from build123d import *

# Parameters (mm, degrees)
SKETCH039_W       = 155
SKETCH039_H       = 187
SKETCH039_R       = 65
PAD004_DEPTH      = 2
PAD005_DEPTH      = 37
SKETCH041_R       = 66
SKETCH041_R_2     = 65
PAD006_DEPTH      = 33
PAD007_DEPTH      = 176
PAD012_DEPTH      = 73.5
PAD012_DEPTH_BACK = 73.5
SKETCH054_W       = 2
SKETCH054_H       = 130
POCKET013_DEPTH   = 2
SKETCH067_R       = 10
POCKET015_DEPTH   = 2
SKETCH068_W       = 7
SKETCH068_H       = 7
SKETCH068_R       = 1.4
PAD022_DEPTH      = 7
POCKET017_DEPTH   = 1
POCKET018_DEPTH   = 1
SKETCH074_R       = 10
POCKET019_DEPTH   = 2
SKETCH075_R       = 1.4
POCKET020_DEPTH   = 2


with BuildPart() as part:
    # Sketch039 → Pad004 (new body)
    with BuildSketch(Plane.XY):
        with Locations((0, -4)):
            Rectangle(SKETCH039_W, SKETCH039_H)
        Circle(SKETCH039_R, mode=Mode.SUBTRACT)
    extrude(amount=PAD004_DEPTH)

    # Sketch040 (on DatumPlane) → Pad005 (join)
    with BuildSketch(Plane.XY.offset(2)):
        Polygon((-77.5, 89.5), (77.5, 89.5), (77.5, -97.5), (75.5, -97.5), (75.5, 87.5), (-75.5, 87.5), (-75.5, -97.5), (-77.5, -97.5), align=None)
    extrude(amount=PAD005_DEPTH)

    # Sketch041 (on DatumPlane) → Pad006 (join)
    with BuildSketch(Plane.XY.offset(2)):
        Circle(SKETCH041_R)
        Circle(SKETCH041_R_2, mode=Mode.SUBTRACT)
    extrude(amount=PAD006_DEPTH)

    # Sketch042 (on DatumPlane) → Pad007 (join)
    with BuildSketch(Plane.XZ.offset(88.5)):
        Polygon((75.5, 29.505045), (75.5, 35), (73.5, 35), align=None)
    pad007 = extrude(amount=-PAD007_DEPTH)

    # Mirrored004: Pad007 across YZ
    add(pad007.mirror(Plane.YZ))

    # Sketch047 → Revolution (revolve)
    with BuildSketch(Plane.XZ):
        Polygon((66, 35), (68, 35), (66, 29.505045), align=None)
    revolve(axis=Axis((0, 0, 0), (0, 0, 1)))

    # Sketch048 → Pad012 (join, two sides)
    with BuildSketch(Plane.YZ) as pad012_sk:
        Polygon((87.5, 35), (87.5, 29.505045), (85.5, 35), align=None)
    extrude(amount=PAD012_DEPTH)
    extrude(pad012_sk.sketch, amount=-PAD012_DEPTH_BACK)

    # Sketch054 → Pocket013 (cut)
    with BuildSketch(Plane.XY):
        with Locations((74.5, 0)):
            Rectangle(SKETCH054_W, SKETCH054_H)
    pocket013 = extrude(amount=POCKET013_DEPTH, mode=Mode.SUBTRACT)

    # Mirrored007: Pocket013 across Sketch054 V_Axis
    add(pocket013.mirror(Plane(origin=(0, 0, 0), x_dir=(0, 0, 1), z_dir=(1, 0, 0))), mode=Mode.SUBTRACT)

    # Sketch067 (on DatumPlane) → Pocket015 (cut)
    with BuildSketch(Plane.XZ.offset(-89.5)):
        with Locations((37.75, 18.5)):
            Circle(SKETCH067_R)
    extrude(amount=POCKET015_DEPTH, mode=Mode.SUBTRACT)

    # Sketch068 (on DatumPlane) → Pad022 (join)
    with BuildSketch(Plane.XZ.offset(97.5)):
        with Locations((-72, 5.5)):
            Rectangle(SKETCH068_W, SKETCH068_H)
        with Locations((-72, 5.5)):
            Circle(SKETCH068_R, mode=Mode.SUBTRACT)
        Polygon((-68.5, 28), (-68.5, 35), (-75.5, 35), (-75.5, 21), align=None)
        with Locations((-72, 31.5)):
            Circle(SKETCH068_R, mode=Mode.SUBTRACT)
    pad022 = extrude(amount=-PAD022_DEPTH)

    # Mirrored009: Pad022 across Sketch068 V_Axis
    add(pad022.mirror(Plane(origin=(0, -97.5, 0), x_dir=(0, -1, 0), z_dir=(1, 0, 0))))

    # Sketch070 (on DatumPlane) → Pocket017 (cut)
    with BuildSketch(Plane.XZ.offset(-89.5)):
        with BuildLine():
            ThreePointArc((44.821068, 11.428932), (37.75, 28.5), (30.678932, 11.428932))
            Line((30.678932, 11.428932), (29.264719, 10.014719))
            ThreePointArc((46.235271, 10.014709), (37.750007, 30.5), (29.264719, 10.014719))
            Line((44.821068, 11.428932), (46.235271, 10.014709))
        make_face()
    extrude(amount=POCKET017_DEPTH, mode=Mode.SUBTRACT)

    # Sketch073 (on DatumPlane) → Pocket018 (cut)
    with BuildSketch(Plane.YZ.offset(77.5)):
        with BuildLine():
            ThreePointArc((2.071068, 11.428932), (-5, 28.5), (-12.071068, 11.428932))
            Line((-13.485281, 10.014719), (-12.071068, 11.428932))
            ThreePointArc((3.485291, 10.014728), (-5.000007, 30.5), (-13.485281, 10.014719))
            Line((2.071068, 11.428932), (3.485291, 10.014728))
        make_face()
    pocket018 = extrude(amount=-POCKET018_DEPTH, mode=Mode.SUBTRACT)

    # Sketch074 (on DatumPlane) → Pocket019 (cut)
    with BuildSketch(Plane.YZ.offset(77.5)):
        with Locations((-5, 18.5)):
            Circle(SKETCH074_R)
    pocket019 = extrude(amount=-POCKET019_DEPTH, mode=Mode.SUBTRACT)

    # Mirrored011: Pocket019 across YZ
    add(pocket019.mirror(Plane.YZ), mode=Mode.SUBTRACT)

    # Mirrored012: Pocket018 across YZ
    add(pocket018.mirror(Plane.YZ), mode=Mode.SUBTRACT)

    # Sketch075 (on DatumPlane) → Pocket020 (cut)
    with BuildSketch(Plane.YZ.offset(77.5)):
        with Locations((-89.5, 18.5)):
            Circle(SKETCH075_R)
        with Locations((79.5, 18.5)):
            Circle(SKETCH075_R)
    pocket020 = extrude(amount=-POCKET020_DEPTH, mode=Mode.SUBTRACT)

    # Mirrored013: Pocket020 across YZ
    add(pocket020.mirror(Plane.YZ), mode=Mode.SUBTRACT)


with BuildPart() as part_1:
    # Body004 placement: moved
    add(part.part.moved(Location((0, 0, -35))))


solid = part_1.part
Could you check a few things on this model? Use its own coordinates, in mm. A direction names the side the tool comes from. Coordinates: 2 decimals unless noted, no trailing zeros. Answer in a Markdown table with one row per item. Add a question column.
(1) I need wall thicknesses on L1, parallel to X at y = 1, z = -26.5; L2, parallel to X at y = -68, z = -7.5; L3, parallel to X at y = 89, z = -16. Which ranges of each line are inside material? Lowest first, please.
(2) If we mould it in two halves opening along Z, with no side actions, what happens to faces 1 (the face through (77.007, -4.604, -4.507)), 2 (the face through (-73, -90.5, -5)), 3 (the face through (72, -94, -10.5)), 4 (the face through (72, -94, 0))? For each: released by +Z, released by -Z, zero draft, split by the parting line, or undercut.
(3) On a 3-axis mill with a long thin cutter (end or side, diameter ignored), from which of +Z, -Z, +X, -X, +Y, -Y can I reach the whole of each face in a straight line? I mean faces 5 (the face through (76.5, -4, -6)), 6 (the face through (39, 88.5, -6)), 7 (the face through (68.5, -94, -30)), 8 (the face through (-72, -94, -10.5)), 9 (the face through (-74.486, -1.732, -2.709)). Say none if no direction works.
(4) If we section it at A-A, the plane x = 41.5: State how many separate pieces and enclosed holes the cut face has, then the cut area to 3 significant figures.
(5) Will these pins go through, and if not, where does the flat tip stop? pin 1 (16.5 mm diameter, centred on y = -9.5, z = -10, fed in from -X); pin 2 (2 mm diameter, centred on x = -72, z = -3.5, fed in from -Y); pin 3 (6 mm diameter, centred on x = 15.5, y = -77.5, fed in from +Z); pin 4 (12 mm diameter, centred on x = -56.5, z = -20.5, fed in from -Y).
Results are:
| question | item | result |
|---|---|---|
| 1 | L1 | x = -77.5 to -75.5, -65.99 to -64.99, 64.99 to 65.99, 75.5 to 77.5 |
| 1 | L2 | x = -77.5 to -75.5, 75.5 to 77.5 |
| 1 | L3 | x = -77.5 to 25.76, 49.74 to 77.5 |
| 2 | face 1 | undercut |
| 2 | face 2 | zero draft |
| 2 | face 3 | undercut |
| 2 | face 4 | released by +Z |
| 3 | face 5 | +X |
| 3 | face 6 | +Y |
| 3 | face 7 | +Z, -Y |
| 3 | face 8 | -Y |
| 3 | face 9 | none |
| 4 | separate pieces | 3 |
| 4 | enclosed holes | 0 |
| 4 | area | 314 mm2 |
| 5 | pin 1 | stops at x = -77.5 |
| 5 | pin 2 | stops at y = 86.41 |
| 5 | pin 3 | stops at z = -33 |
| 5 | pin 4 | stops at y = -42.49 |
